Design review of the part shown in the three views and the two pictorial views. Dimensions are in mm from the part's minimum x, y and z. A direction names the side the tool comes from. Give positions to 0.01 mm unless a question says otherwise; leave off trailing zeros. Order: outer loops, then holes, each group sorted by start corner. A loop starts at its lowest first (then second) coordinate and runs counter-clockwise, first axis right, second up.
Item 1: Machinability: for the marked faces 1 and 2, which of the approach directions +Z, -Z, +X, -X, +Y, -Y give a long, thin tool a straight path to every point of the face, cutting with its end or side? Answer none if there is none.
Item 2: Consider section D-D (z = 33). Give the boundary of the cut face in (x, y).
Item 3: For probe 1 along Z at (x, y) = (26.5, 30.5) (1 decimal); probe 2 along X at (y, z) = (12, 14) (1 decimal); probe 3 along X at (y, z) = (19, 12.7), list the stretches that pass through material, from the lowest coordinate up.
Item 4: Consider section C-C (y = 14). Give the boundary of the cut face in (x, z) (1 decimal), plus the area to 3 significant figures.
Item 5: The part is to be moulded in two halves that separate along X. For the marked faces 3, 4 and 5, say which applies: released by +X, released by -X, zero draft, split by the parting line, or undercut.
Item 6: Consider section B-B (z = 38.1). Give the boundary of the cut face in (x, y), plus the area to 3 significant figures.
Item 7: For P1, Ø4, axis at x = 18, y = 28.5, coming from the +Z side; P2, Ø5, axis at x = 43, y = 29, coming from the +Z side (1 decimal); P3, Ø10, axis at y = 21.5, z = 8, coming from the -X side, all flat-tipped, find the tip position at first contact; note any pin that passes through.
Item 8: Consider section A-A (x = 25.4). Give the boundary of the cut face in (y, z).
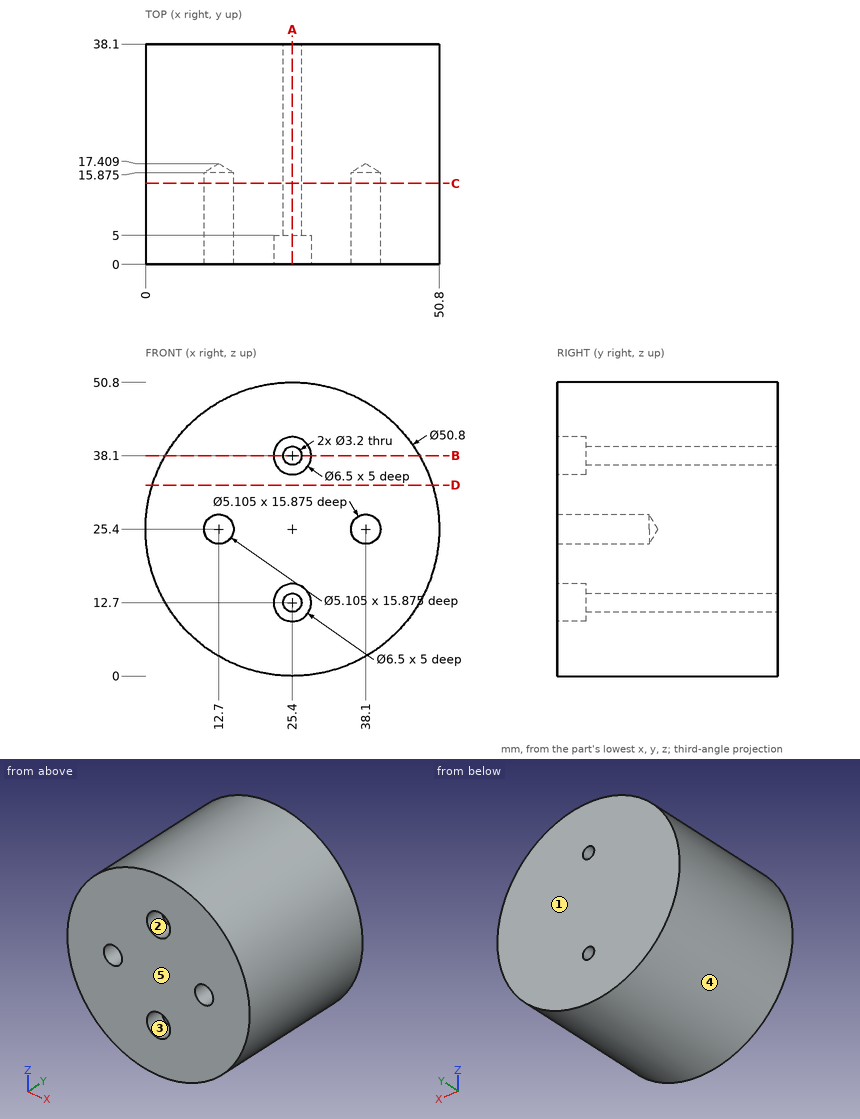
Resolved:
1. face 1: +Z, -Z, +X, -X, +Y
1. face 2: -Y
2. outline: (1.16, 0) - (49.64, 0) - (49.64, 38.1) - (1.16, 38.1) - close
3. probe 1: z = 0 to 11.5, 13.9 to 36.9, 39.3 to 50.8
3. probe 2: x = 2.7 to 24.5, 26.3 to 48.1
3. probe 3: x = 3.4 to 23.8, 27 to 47.4
4. outline: circle Ø50.8 at (25.4, 25.4); hole circle Ø5.1 at (12.7, 25.4); hole circle Ø3.2 at (25.4, 12.7); hole circle Ø3.2 at (25.4, 38.1); hole circle Ø5.1 at (38.1, 25.4)
4. area: 1,970 mm2
5. face 3: undercut
5. face 4: split by the parting line
5. face 5: zero draft
6. outline: (3.4, 0) - (22.15, 0) - (22.15, 5) - (23.8, 5) - (23.8, 38.1) - (3.4, 38.1) - close; (27, 5) - (28.65, 5) - (28.65, 0) - (47.4, 0) - (47.4, 38.1) - (27, 38.1) - close
6. area: 1,540 mm2
7. P1: stops at z = 50.22
7. P2: stops at z = 45.8
7. P3: stops at x = 3.23
8. outline: (0, 0) - (38.1, 0) - (38.1, 11.1) - (5, 11.1) - (5, 9.45) - (0, 9.45) - close; (0, 15.95) - (5, 15.95) - (5, 14.3) - (38.1, 14.3) - (38.1, 36.5) - (5, 36.5) - (5, 34.85) - (0, 34.85) - close; (0, 41.35) - (5, 41.35) - (5, 39.7) - (38.1, 39.7) - (38.1, 50.8) - (0, 50.8) - close
